Could you check a few things on this model? Use its own coordinates, in mm. A direction names the side the tool comes from. Round coordinates to 2 decimals unless told otherwise and drop trailing zeros. Loops run counter-clockwise (first coordinate to the right, second up) from the corner with the lowest first, then second, coordinate; pieces in that order, holes last. Notation, with made-up numbers: (-23, 53.25) -> (-9, 53.25) arc R32 cw to (-9, 90.25) -> close; hole circle Ø8 at (82.5, 85). An arc over 180 degrees is marked (long way). Use CSV: the item, a comma, the result in double quotes. Start each with the question number.
Autodesk Inventor part; units mm, degrees
ref_plane "YZ Plane" through (0, 0, 0) normal (1, 0, 0) x (0, 1, 0)
ref_plane "XZ Plane" through (0, 0, 0) normal (0, 1, 0) x (-1, 0, 0)
ref_plane "XY Plane" through (0, 0, 0) normal (0, 0, 1) x (1, 0, 0)
sketch "Sketch1" plane through (0, 0, 0) normal (0, 0, 1) x (1, 0, 0)
  circle A0 centre (0, 0) radius 5
  dimension "d0" = 10
extrude "Extrusion1" add sketch "Sketch1" against normal blind 175
ref_plane "Work Plane1" through (0, 0, -100) normal (0, 0, 1) x (1, 0, 0)
sketch "Sketch2" plane through (0, 0, 0) normal (0, 1, 0) x (-1, 0, 0)
  circle A0 centre (0, -137.5) radius 5
  line L0 (-5, -175) -> (5, -175)
  point P0 (0, 0)
  dimension "d4" = 10
  dimension "d5" = 37.5
extrude "Extrusion2" add sketch "Sketch2" along normal mid plane 75
sketch "Sketch5" plane through (0, 0, -100) normal (0, 0, 1) x (1, 0, 0)
  line L0 (5, 37.5) -> (-5, 37.5)
  arc A0 (-5, 37.5) -> (-18.5426, 95.9905) centre (-137.4066, 37.6564) ccw
  arc A1 (5, 37.5) -> (-14.4042, 96.255) centre (-129.1845, 25.7664) ccw
  arc A2 (-14.4042, 96.255) -> (-18.5426, 95.9905) centre (-16.4034, 95.0273) ccw
  line L1 (-5, -37.5) -> (5, -37.5)
  arc A3 (5, -37.5) -> (17.351, -93.4908) centre (120.393, -41.4031) ccw
  arc A4 (-5, -37.5) -> (13.2332, -94.5364) centre (105.5133, -33.604) ccw
  line L2 (5, -37.5) -> (-5, -37.5)
  line L3 (5, 37.5) -> (-5, 37.5)
  arc A5 (13.2332, -94.5364) -> (17.351, -93.4908) centre (15.1102, -93.297) ccw
  point P0 (0, 0)
extrude "Extrusion4" add sketch "Sketch5" against normal blind 75
properties part number "wet_proj_aandrijstang_2"
1. Suppose I cut it at D-D (y = -56). List the corners of the cut face in (x, z) for me, then the cut area to 3 significant figures.
2. We'd pull the mould along Y, two halves only. Please class faces 1 (the face through (0.054, -66.871, -136.975)), 2 (the face through (-16.52, 97.37, -136.98)), 3 (the face through (4.77, 1.5, -67.79)), 4 (the face through (0, -37.5, -156)): pulls with the +Y half, pulls with the -Y half, needs draft (parallel to the pull), parting line crosses it, or undercut.
3. If I drill on L1, parallel to Z at x = 6, y = -66.5; L2, parallel to Y at x = -15, z = -142; L3, parallel to Z at x = -3.5, y = -37, over which ranges is the centre line in solid material (lowest first)?
4. Suppose I cut it at A-A (x = 0). List the corners of the cut face in (y, z) for me.
5. Suppose I cut it at C-C (z = -44). List the corners of the cut face in (x, y) for me.
6. Will these pins go through, and if not, where does the flat tip stop? pin 1 (4 mm diameter, centred on x = 2, z = -100.5, fed in from -Y); pin 2 (12 mm diameter, centred on x = 6.5, y = -44.5, fed in from +Z); pin 3 (6 mm diameter, centred on x = -4.5, y = -69.5, fed in from -Z); pin 4 (8 mm diameter, centred on y = -37, z = -127, fed in from -X).
7. For faces 5 (the face through (-0.651, 4.957, -155.988)), 6 (the face through (4, -64, -100)), 7 (the face through (0.651, -18.488, -132.543)), which set-ups out of +Z, -Z, +X, -X, +Y, -Y let a thin tool reach every point of the face, with its end or its side?
8. Suppose I cut it at B-B (y = 23). List the corners of the cut face in (x, z) for me.
Geometry check:
1,outline,"(-2.78, -175) -> (5.86, -175) -> (5.86, -100) -> (-2.78, -100) -> close"
1,area,"648 mm²"
2,face 1,"pulls with the -Y half"
2,face 2,"pulls with the +Y half"
2,face 3,"undercut"
2,face 4,"undercut"
3,L1,"z = -175 to -100"
3,L2,"y = 88.14 to 96.91"
3,L3,"z = -141.07 to -133.93"
4,outline,"(-66.7, -175) -> (-37.5, -175) -> (-37.5, -142.5) -> (-5, -142.5) -> (-5, -175) -> (5, -175) -> (5, -142.5) -> (37.5, -142.5) -> (37.5, -175) -> (63.9, -175) -> (63.9, -100) -> (37.5, -100) -> (37.5, -132.5) -> (5, -132.5) -> (5, 0) -> (-5, 0) -> (-5, -132.5) -> (-37.5, -132.5) -> (-37.5, -100) -> (-66.7, -100) -> close"
5,outline,"circle Ø10 at (0, 0)"
6,pin 1,"stops at y = -77.46"
6,pin 2,"stops at z = -100"
6,pin 3,"passes through"
6,pin 4,"stops at x = -5"
7,face 5,"-Z"
7,face 6,"+Z, +X, -X, -Y"
7,face 7,"none"
8,outline,"circle Ø10 at (0, -137.5)"
